Source: CAD feature listing. Evaluate the final solid. Frame: model axes, mm. A direction names the side the tool comes from. Give positions to 0.01 mm unless a question says otherwise; leave off trailing zeros. Loops run counter-clockwise (first coordinate to the right, second up) from the corner with the lowest first, then second, coordinate; pieces in that order, holes last. Notation, with made-up numbers: M 44,89 L 74,89 A19 ccw 74,116 Z; hole C 71.5,33 d9. An arc over 180 degrees is marked long. Answer in a Markdown table with one row per item.
```python
from build123d import *

# Parameters (mm, degrees)
F0_W     = 100
F0_H     = 100
F1_DEPTH = 100
F3_SIZE  = 25
F4_SIZE  = 25
F5_DEPTH = 100


with BuildPart() as f1:
    # F0 (on Front) → F1 (new body)
    with BuildSketch(Plane.XZ):
        with Locations((14.669374, 9.856632)):
            Rectangle(F0_W, F0_H)
    extrude(amount=F1_DEPTH)

    # F3
    f3_edges = [f1.edges().sort_by_distance(p)[0] for p in [
        (64.669374, -50, 59.856632),
    ]]
    chamfer(f3_edges, length=F3_SIZE)

    # F4
    f4_edges = [f1.edges().sort_by_distance(p)[0] for p in [
        (-35.330626, -50, -40.143368),
    ]]
    chamfer(f4_edges, length=F4_SIZE)

    # F2 (on face) → F5 (cut)
    with BuildSketch(Plane.XZ.offset(100)):
        Polygon((15, 17.688339), (0, 43.669101), (-15, 17.688339), align=None)
    extrude(amount=-F5_DEPTH, mode=Mode.SUBTRACT)


solid = f1.part
```
Q1. Mould query, pull axis X, two halves, no side actions, for faces 3 (the flat face through (-7.395, -50.7, 30.861)), 4 (the flat face through (-23.006, -49.3, -27.468)), 5 (the flat face through (64.669, -49, -3)). Classes: +X half, -X half, draft (parallel to the pull), parting line (faces both ways), or undercut.
Values follow:
| item | result |
|---|---|
| face 3 | undercut |
| face 4 | -X half |
| face 5 | +X half |
Q2. Reachability of faces 1 (the flat face through (-35.331, -49, 22)), 2 (the flat face through (7.605, -50.7, 30.497)) from +Z, -Z, +X, -X, +Y, -Y: full face, straight path, thin tool, end or side. Return the list, or none.
Values follow:
| item | result |
|---|---|
| face 1 | +Z, -Z, -X, +Y, -Y |
| face 2 | +Y, -Y |
Q3. Ray query, probe 1 along X at (y, z) = (-81.5, 31); probe 2 along Z at (x, y) = (11, -61); probe 3 along X at (y, z) = (-46, 30.5). Return the intervals inside material, ascending. Write a range as from..to.
Values follow:
| item | result |
|---|---|
| probe 1 | -35.33..-7.31, 7.31..64.67 |
| probe 2 | -40.14..17.69, 24.62..59.86 |
| probe 3 | -35.33..-7.6, 7.6..64.67 |
Q4. Section query A-A (x = 2). Output: boundary loops of the cut face in (y, z) (3 decimals).
Values follow:
| item | result |
|---|---|
| outline | M -100,-40.143 L 0,-40.143 L 0,17.688 L -100,17.688 Z; M -100,40.205 L 0,40.205 L 0,59.857 L -100,59.857 Z |
Q5. Section query B-B (y = -68). Output: boundary loops of the cut face in (x, z).
Values follow:
| item | result |
|---|---|
| outline | M -35.33,-15.14 L -10.33,-40.14 L 64.67,-40.14 L 64.67,34.86 L 39.67,59.86 L -35.33,59.86 Z; hole M -15,17.69 L 15,17.69 L 0,43.67 Z |
Q6. Section query C-C (z = 23.5). Output: boundary loops of the cut face in (x, y).
Values follow:
| item | result |
|---|---|
| outline | M -35.33,-100 L -11.64,-100 L -11.64,0 L -35.33,0 Z; M 11.64,-100 L 64.67,-100 L 64.67,0 L 11.64,0 Z |
Q7. Section query D-D (x = -19). Output: boundary loops of the cut face in (y, z).
Values follow:
| item | result |
|---|---|
| outline | M -100,-31.47 L 0,-31.47 L 0,59.86 L -100,59.86 Z |
